from build123d import *

# Parameters (mm, degrees)
F0_W     = 76.2
F0_H     = 76.2
F3_DEPTH = 6.35
F4_DEPTH = 6.351
F2_R     = 2.794
F5_DEPTH = 6.351
F6_W     = 9.525
F6_H     = 9.525
F6_R     = 2.032
F7_DEPTH = 9.525


with BuildPart() as f3:
    # F0 (on Front) → F3 (new body)
    with BuildSketch(Plane.XZ):
        Rectangle(F0_W, F0_H)
    extrude(amount=F3_DEPTH)

    # F1 (on Front) → F4 (cut, through all)
    with BuildSketch(Plane.XZ):
        with BuildLine():
            Line((21.336, 22.606), (-21.336, 22.606))
            ThreePointArc((-21.336, 22.606), (-23.504026, 23.504026), (-22.606, 21.336))
            Line((-22.606, 21.336), (-22.606, -21.336))
            ThreePointArc((-22.606, -21.336), (-23.504026, -23.504026), (-21.336, -22.606))
            Line((-21.336, -22.606), (21.336, -22.606))
            ThreePointArc((21.336, -22.606), (23.504026, -23.504026), (22.606, -21.336))
            Line((22.606, -21.336), (22.606, 21.336))
            ThreePointArc((22.606, 21.336), (23.504026, 23.504026), (21.336, 22.606))
        make_face()
    extrude(amount=F4_DEPTH, mode=Mode.SUBTRACT)

    # F2 (on Front) → F5 (cut, through all)
    with BuildSketch(Plane.XZ):
        with Locations((-31.75, 31.75)):
            Circle(F2_R)
        with Locations((-31.75, -31.75)):
            Circle(F2_R)
        with Locations((31.75, -31.75)):
            Circle(F2_R)
        with Locations((31.75, 31.75)):
            Circle(F2_R)
    extrude(amount=F5_DEPTH, mode=Mode.SUBTRACT)

    # F6 (on face) → F7 (join)
    with BuildSketch(Plane.XY.offset(38.1)):
        with Locations((-19.05, 4.7625)):
            Rectangle(F6_W, F6_H)
        with Locations((-19.05, 4.7625)):
            Circle(F6_R, mode=Mode.SUBTRACT)
        with Locations((19.05, 4.7625)):
            Rectangle(F6_W, F6_H)
        with Locations((19.05, 4.7625)):
            Circle(F6_R, mode=Mode.SUBTRACT)
    extrude(amount=-F7_DEPTH)


solid = f3.part
Model file for the job. Use its own axes, mm. A direction names the side the tool comes from. Coordinates: 2 decimals unless noted, no trailing zeros. Order: outer loops, then holes, each group sorted by start corner. A loop starts at its lowest first (then second) coordinate and runs counter-clockwise, first axis right, second up. Notation, with made-up numbers: (85.5, 12) -> (114.5, 12) arc R21 ccw to (114.5, 46) -> close; hole circle Ø7 at (32, 44). An arc over 180 degrees is marked (long way). Return JSON: item names as keys, results as strings. Group by question number.
Item 1: Saw through at C-C on x = 3.5. Write the cut outline in (y, z), then the cut area to 3 significant figures.
Item 2: Saw through at A-A on z = 30. State how many separate pieces and enclosed holes the cut face has, then the cut area to 3 significant figures.
Item 3: Flat gauge pins, fed straight in: P1, Ø3.5, axis at x = 22.606, z = -22.606, coming from the +Y side; P2, Ø5, axis at y = 3.5, z = 31.5, coming from the -X side. Where does each tip first touch, or does it go through?
Item 4: Pull direction Y, two halves, no side cores. Call faces 1 (the cylindrical face through (-20.663, 3.526, 33.404)), 2 (the flat face through (0, -3, 22.606)), 3 (the flat face through (19, 9.525, 33)): pulls with the +Y half, pulls with the -Y half, needs draft (parallel to the pull), parting line crosses it, or undercut.
Item 5: Wall check: line 1 along X through (y, z) = (-5, -31.75); line 2 along Z through (x, y) = (-7.5, -2.25). Give the ranges that are in metal, low to high. Write a range as [from, to].
Item 6: Saw through at D-D on y = -2.25. Write the cut outline in (x, z), then the cut area to 3 significant figures.
Item 7: Saw through at B-B on z = -15. Write the cut outline in (x, y).
Item 8: Tool access for faces 4 (the flat face through (22.606, -3, 0)), 5 (the flat face through (-21.233, 4.829, 28.575)), 6 (the flat face through (23.812, 5, 33)), 7 (the flat face through (-23.812, 5, 33)): list every direction of +Z, -Z, +X, -X, +Y, -Y with a clear straight run to the whole face (end or side of a thin tool).
Values found:
{
 "1": {"outline": "(-6.35, -38.1) -> (0, -38.1) -> (0, -22.61) -> (-6.35, -22.61) -> close; (-6.35, 22.61) -> (0, 22.61) -> (0, 38.1) -> (-6.35, 38.1) -> close", "area": "197 mm2"},
 "2": {"separate pieces": "3", "enclosed holes": "2", "area": "584 mm2"},
 "3": {"P1": "stops at y = 0", "P2": "stops at x = -23.81"},
 "4": {"face 1": "undercut", "face 2": "needs draft", "face 3": "pulls with the +Y half"},
 "5": {"line 1": "x = [-38.1, -34.54], [-28.96, 28.96], [34.54, 38.1]", "line 2": "z = [-38.1, -22.61], [22.61, 38.1]"},
 "6": {"outline": "(-38.1, -38.1) -> (38.1, -38.1) -> (38.1, 38.1) -> (-38.1, 38.1) -> close; hole circle Ø5.59 at (-31.75, -31.75); hole circle Ø5.59 at (-31.75, 31.75); hole (-22.61, -21.34) arc R1.27 ccw (long way) to (-21.34, -22.61) -> (21.34, -22.61) arc R1.27 ccw (long way) to (22.61, -21.34) -> (22.61, 21.34) arc R1.27 ccw (long way) to (21.34, 22.61) -> (-21.34, 22.61) arc R1.27 ccw (long way) to (-22.61, 21.34) -> close; hole circle Ø5.59 at (31.75, -31.75); hole circle Ø5.59 at (31.75, 31.75)", "area": "3,650 mm2"},
 "7": {"outline": "(-38.1, -6.35) -> (-22.61, -6.35) -> (-22.61, 0) -> (-38.1, 0) -> close; (22.61, -6.35) -> (38.1, -6.35) -> (38.1, 0) -> (22.61, 0) -> close"},
 "8": {"face 4": "+Y, -Y", "face 5": "-Z, +X, -X, +Y", "face 6": "+Z, -Z, +X, +Y", "face 7": "+Z, -Z, -X, +Y"}
}
